Model file for the job. Use its own axes, mm. Give positions to 0.01 mm unless a question says otherwise; leave off trailing zeros. Loops run counter-clockwise (first coordinate to the right, second up) from the corner with the lowest first, then second, coordinate; pieces in that order, holes last. Notation, with made-up numbers: M 62.5,36.5 L 115.5,36.5 A31 ccw 115.5,63.5 Z; hole C 3.25,66.5 d3. An arc over 180 degrees is marked long. Answer in a Markdown table with one row per item.
```python
from build123d import *

# Parameters (mm, degrees)
SKIZZE1_W                       = 45
SKIZZE1_H                       = 85
AUFSATZ_LINEAR_AUSTRAGEN1_DEPTH = 5
SKIZZE6_R                       = 1.6
SCHNITT_LINEAR_AUSTRAGEN2_DEPTH = 3
SKIZZE7_W                       = 37
SKIZZE7_H                       = 1.7
SCHNITT_LINEAR_AUSTRAGEN3_DEPTH = 10
SKIZZE8_W                       = 31
SKIZZE8_H                       = 38.15
SCHNITT_LINEAR_AUSTRAGEN4_DEPTH = 10
SKIZZE9_W                       = 38.051320542
SKIZZE9_H                       = 40.768170305
AUFSATZ_LINEAR_AUSTRAGEN2_DEPTH = 2


with BuildPart() as part:
    # Skizze1 → Aufsatz-Linear austragen1 (new body)
    with BuildSketch(Plane.XY):
        with Locations((22.5, 42.5)):
            Rectangle(SKIZZE1_W, SKIZZE1_H)
    extrude(amount=AUFSATZ_LINEAR_AUSTRAGEN1_DEPTH)

    # Skizze6 → Schnitt-Linear austragen2 (cut)
    with BuildSketch(Plane.XY.offset(5)):
        with Locations((6, 80)):
            Circle(SKIZZE6_R)
        with Locations((39, 80)):
            Circle(SKIZZE6_R)
        with Locations((39, 5)):
            Circle(SKIZZE6_R)
        with Locations((6, 5)):
            Circle(SKIZZE6_R)
    extrude(amount=-SCHNITT_LINEAR_AUSTRAGEN2_DEPTH, mode=Mode.SUBTRACT)

    # Skizze7 → Schnitt-Linear austragen3 (cut)
    with BuildSketch(Plane.XY.offset(5)):
        with Locations((22.5, 58.8)):
            Rectangle(SKIZZE7_W, SKIZZE7_H)
        with Locations((22.5, 54.75)):
            Rectangle(SKIZZE7_W, SKIZZE7_H)
        with Locations((22.5, 50.7)):
            Rectangle(SKIZZE7_W, SKIZZE7_H)
        with Locations((22.5, 46.65)):
            Rectangle(SKIZZE7_W, SKIZZE7_H)
        with Locations((22.5, 42.6)):
            Rectangle(SKIZZE7_W, SKIZZE7_H)
        with Locations((22.5, 38.55)):
            Rectangle(SKIZZE7_W, SKIZZE7_H)
        with Locations((22.5, 34.5)):
            Rectangle(SKIZZE7_W, SKIZZE7_H)
        with Locations((22.5, 30.45)):
            Rectangle(SKIZZE7_W, SKIZZE7_H)
        with Locations((22.5, 26.4)):
            Rectangle(SKIZZE7_W, SKIZZE7_H)
        with Locations((22.5, 22.35)):
            Rectangle(SKIZZE7_W, SKIZZE7_H)
    extrude(amount=-SCHNITT_LINEAR_AUSTRAGEN3_DEPTH, mode=Mode.SUBTRACT)

    # Skizze8 → Schnitt-Linear austragen4 (cut)
    with BuildSketch(Plane.XY.offset(5)):
        with Locations((22.5, 40.575)):
            Rectangle(SKIZZE8_W, SKIZZE8_H)
    extrude(amount=-SCHNITT_LINEAR_AUSTRAGEN4_DEPTH, mode=Mode.SUBTRACT)

    # Skizze9 → Aufsatz-Linear austragen2 (add)
    with BuildSketch(Plane(origin=(0, 0, 0), x_dir=(-1, 0, 0), z_dir=(0, 0, -1))):
        with Locations((-22.316575494, 40.457263066)):
            Rectangle(SKIZZE9_W, SKIZZE9_H)
    extrude(amount=-AUFSATZ_LINEAR_AUSTRAGEN2_DEPTH)


solid = part.part
```
Q1. Mould opens along Y. For faces 1 (the face through (6, 5, 2)), 2 (the face through (22, 85, 2)) say: released by +Y, released by -Y, zero draft, split by the parting line, or undercut.
Reported:
| item | result |
|---|---|
| face 1 | undercut |
| face 2 | released by +Y |
Q2. Saw through at D-D (z = 3.85). Give the number of separate pieces and of enclosed holes in the cut face, and give its area (3 significant figures).
Reported:
| item | result |
|---|---|
| separate pieces | 1 |
| enclosed holes | 5 |
| area | 2,510 mm² |
Q3. Probe probe 1 along X at (y, z) = (80, 4.15); probe 2 along Y at (x, z) = (34, 4.5); probe 3 along X at (y, z) = (46, 3.75). List the from-to ranges inside material, lowest first.
Reported:
| item | result |
|---|---|
| probe 1 | 0 to 4.4, 7.6 to 37.4, 40.6 to 45 |
| probe 2 | 0 to 21.5, 59.65 to 85 |
| probe 3 | 0 to 4, 41 to 45 |
Q4. Saw through at A-A (x = 35). Give the cut face in (y, z).
Reported:
| item | result |
|---|---|
| outline | M 0,0 L 85,0 L 85,5 L 59.65,5 L 59.65,2 L 21.5,2 L 21.5,5 L 0,5 Z |
Q5. Saw through at B-B (y = 52.5). Give the cut face in (x, z).
Reported:
| item | result |
|---|---|
| outline | M 0,0 L 45,0 L 45,5 L 38,5 L 38,2 L 7,2 L 7,5 L 0,5 Z |
Q6. Saw through at C-C (y = 5). Give the cut face in (x, z), and give its area (3 significant figures).
Reported:
| item | result |
|---|---|
| outline | M 0,0 L 45,0 L 45,5 L 40.6,5 L 40.6,2 L 37.4,2 L 37.4,5 L 7.6,5 L 7.6,2 L 4.4,2 L 4.4,5 L 0,5 Z |
| area | 206 mm² |
